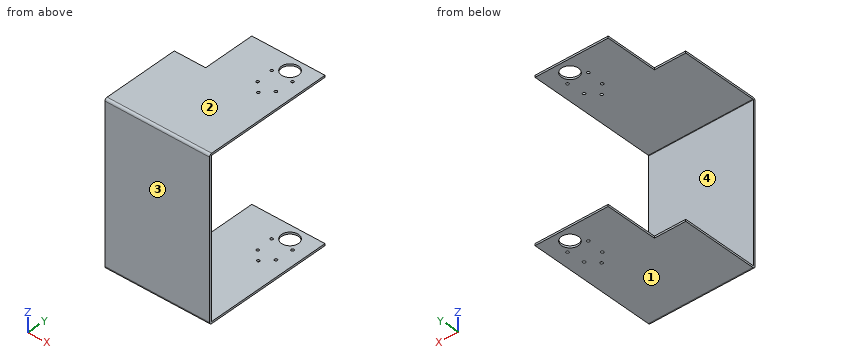
Autodesk Inventor part; units mm, degrees
ref_plane "YZ Plane" through (0, 0, 0) normal (1, 0, 0) x (0, 1, 0)
ref_plane "XZ Plane" through (0, 0, 0) normal (0, 1, 0) x (-1, 0, 0)
ref_plane "XY Plane" through (0, 0, 0) normal (0, 0, 1) x (1, 0, 0)
sketch "Sketch1" plane through (0, 0, 0) normal (0, 1, 0) x (-1, 0, 0)
  line L0 (0, 0) -> (80, 0)
  line L1 (80, 0) -> (80, 120)
  line L2 (80, 120) -> (0, 120)
  line L3 (0, 120) -> (0, 0)
  dimension "d0" = 80
  dimension "d1" = 120
extrude "Plate1" add sketch "Sketch1" along normal blind 1.5
sketch "Sketch2" plane through (0, 0, 121.5) normal (0, 0, -1) x (-1, 0, 0)
  line L0 (80, 0) -> (0, 0)
  line L1 (0, 0) -> (0, 100)
  line L2 (0, 100) -> (80, 100)
  line L3 (80, 100) -> (80, 0)
edge flange "Flange1" height 100 angle 90 thickness 1.5 bend radius 0.31 thickness toward (0, 0, -1) relief tear relief width 1.5 relief depth 0.75 edges at (-40, 1.5, 120) wall of the first edge with corners at (-80, 0, 121.5) (0, 0, 121.5) (0, 100, 121.5) (-80, 100, 121.5)
bend "Bend1"
corner "Corner1"
sketch "Sketch3" plane through (-80, 0, -1.5) normal (0, 0, 1) x (1, 0, 0)
  line L0 (80, 0) -> (0, 0)
  line L1 (0, 0) -> (0, 100)
  line L2 (0, 100) -> (80, 100)
  line L3 (80, 100) -> (80, 0)
edge flange "Flange2" height 100 angle 90 thickness 1.5 bend radius 0.31 thickness toward (0, 0, 1) relief tear relief width 1.5 relief depth 0.75 edges at (-40, 1.5, 0) wall of the first edge with corners at (0, 0, -1.5) (-80, 0, -1.5) (-80, 100, -1.5) (0, 100, -1.5)
bend "Bend2"
corner "Corner2"
sketch "Sketch4" plane through (0, 100, -1.5) normal (0, 0, -1) x (-1, 0, 0)
  line L0 (56, -40) -> (80, -40)
  line L1 (80, -40) -> (80, 0)
  line L2 (80, 0) -> (56, 0)
  line L3 (56, 0) -> (56, -40)
  line L4 (80, 0) -> (80, -98.19)
  line L5 (0, 0) -> (80, 0)
  point P0 (0, -100)
  dimension "d23" = 24
  dimension "d24" = 40
extrude "Cut1" cut sketch "Sketch4" against normal blind 1.5
sketch "Sketch5" plane through (0, 100, 120) normal (0, 0, -1) x (-1, 0, 0)
  point P0 (0, -100)
sketch "Sketch6" plane through (-80, 100, 121.5) normal (0, 0, 1) x (1, 0, 0)
  line L0 (24, 0) -> (0, 0)
  line L1 (0, 0) -> (0, -40)
  line L2 (0, -40) -> (24, -40)
  line L3 (24, -40) -> (24, 0)
  line L4 (0, -98.19) -> (0, 0)
  line L5 (0, 0) -> (80, 0)
  point P0 (80, -100)
  dimension "d27" = 40
  dimension "d28" = 24
extrude "Cut2" cut sketch "Sketch6" against normal blind 1.5
sketch "Sketch7" plane through (0, 1.81, -1.5) normal (0, 0, -1) x (-1, 0, 0)
  circle A0 centre (17.93, 60.77) radius 0.7835
  circle A1 centre (10.93, 68.07) radius 0.7835
  circle A2 centre (24.93, 68.07) radius 0.7835
  circle A3 centre (9.93, 81.29) radius 0.7835
  circle A4 centre (25.93, 81.29) radius 0.7835
  line L0 (24, 59.37) -> (11.86, 59.37)
  line L1 (24, 59.37) -> (24, 60.09)
  arc A5 (26, 62.09) -> (24, 60.09) centre (26, 60.09) ccw
  line L2 (26, 62.09) -> (26.72, 62.09)
  line L3 (26.72, 94.19) -> (26.72, 62.09)
  line L4 (26.72, 94.19) -> (26, 94.19)
  arc A6 (24, 96.19) -> (26, 94.19) centre (26, 96.19) ccw
  line L5 (24, 96.19) -> (24, 96.91)
  line L6 (11.86, 96.91) -> (24, 96.91)
  line L7 (11.86, 96.91) -> (11.86, 96.19)
  arc A7 (9.86, 94.19) -> (11.86, 96.19) centre (9.86, 96.19) ccw
  line L8 (9.86, 94.19) -> (9.14, 94.19)
  line L9 (9.14, 62.09) -> (9.14, 94.19)
  line L10 (9.14, 62.09) -> (9.86, 62.09)
  arc A8 (11.86, 60.09) -> (9.86, 62.09) centre (9.86, 60.09) ccw
  line L11 (11.86, 60.09) -> (11.86, 59.37)
  circle A9 centre (17.93, 88.19) radius 6.4
  point P0 (0, -1.81)
  point P1 (11.86, 94.19)
hole "Hole1" at (-10.93, 69.88, -1.5) at (-9.93, 83.1, -1.5) at (-25.93, 83.1, -1.5) at (-24.93, 69.88, -1.5) at (-17.93, 62.58, -1.5) direction (0, 0, 1) diameter 2.1 depth 1.5
sketch "Sketch8" plane through (-80, 1.81, 121.5) normal (0, 0, 1) x (1, 0, 0)
  circle A0 centre (62.07, 60.77) radius 0.7835
  circle A1 centre (55.07, 68.07) radius 0.7835
  circle A2 centre (69.07, 68.07) radius 0.7835
  circle A3 centre (54.07, 81.29) radius 0.7835
  circle A4 centre (70.07, 81.29) radius 0.7835
  line L0 (68.14, 59.37) -> (56, 59.37)
  line L1 (68.14, 59.37) -> (68.14, 60.09)
  arc A5 (70.14, 62.09) -> (68.14, 60.09) centre (70.14, 60.09) ccw
  line L2 (70.14, 62.09) -> (70.86, 62.09)
  line L3 (70.86, 94.19) -> (70.86, 62.09)
  line L4 (70.86, 94.19) -> (70.14, 94.19)
  arc A6 (68.14, 96.19) -> (70.14, 94.19) centre (70.14, 96.19) ccw
  line L5 (68.14, 96.19) -> (68.14, 96.91)
  line L6 (56, 96.91) -> (68.14, 96.91)
  line L7 (56, 96.91) -> (56, 96.19)
  arc A7 (54, 94.19) -> (56, 96.19) centre (54, 96.19) ccw
  line L8 (54, 94.19) -> (53.28, 94.19)
  line L9 (53.28, 62.09) -> (53.28, 94.19)
  line L10 (53.28, 62.09) -> (54, 62.09)
  arc A8 (56, 60.09) -> (54, 62.09) centre (54, 60.09) ccw
  line L11 (56, 60.09) -> (56, 59.37)
  circle A9 centre (62.07, 88.19) radius 6.4
  point P0 (80, -1.81)
  point P1 (56, 94.19)
hole "Hole2" at (-25.93, 83.1, 121.5) at (-9.93, 83.1, 121.5) at (-10.93, 69.88, 121.5) at (-24.93, 69.88, 121.5) at (-17.93, 62.58, 121.5) direction (0, 0, -1) diameter 2.1 depth 1.5
sketch "Sketch9" plane through (-80, 1.81, 121.5) normal (0, 0, 1) x (1, 0, 0)
  circle A0 centre (62.07, 60.77) radius 0.7835
  circle A1 centre (55.07, 68.07) radius 0.7835
  circle A2 centre (69.07, 68.07) radius 0.7835
  circle A3 centre (54.07, 81.29) radius 0.7835
  circle A4 centre (70.07, 81.29) radius 0.7835
  line L0 (68.14, 59.37) -> (56, 59.37)
  line L1 (68.14, 59.37) -> (68.14, 60.09)
  arc A5 (70.14, 62.09) -> (68.14, 60.09) centre (70.14, 60.09) ccw
  line L2 (70.14, 62.09) -> (70.86, 62.09)
  line L3 (70.86, 94.19) -> (70.86, 62.09)
  line L4 (70.86, 94.19) -> (70.14, 94.19)
  arc A6 (68.14, 96.19) -> (70.14, 94.19) centre (70.14, 96.19) ccw
  line L5 (68.14, 96.19) -> (68.14, 96.91)
  line L6 (56, 96.91) -> (68.14, 96.91)
  line L7 (56, 96.91) -> (56, 96.19)
  arc A7 (54, 94.19) -> (56, 96.19) centre (54, 96.19) ccw
  line L8 (54, 94.19) -> (53.28, 94.19)
  line L9 (53.28, 62.09) -> (53.28, 94.19)
  line L10 (53.28, 62.09) -> (54, 62.09)
  arc A8 (56, 60.09) -> (54, 62.09) centre (54, 60.09) ccw
  line L11 (56, 60.09) -> (56, 59.37)
  circle A9 centre (62.07, 88.19) radius 6.4
  circle A10 centre (62.07, 88.19) radius 6.5
  point P0 (80, -1.81)
  point P1 (56, 94.19)
  dimension "d45" = 13
extrude "Extrusion1" cut sketch "Sketch9" against normal blind 1.5 contours A9 | A10
sketch "Sketch10" plane through (0, 1.81, -1.5) normal (0, 0, -1) x (-1, 0, 0)
  circle A0 centre (17.93, 60.77) radius 0.7835
  circle A1 centre (10.93, 68.07) radius 0.7835
  circle A2 centre (24.93, 68.07) radius 0.7835
  circle A3 centre (9.93, 81.29) radius 0.7835
  circle A4 centre (25.93, 81.29) radius 0.7835
  line L0 (24, 59.37) -> (11.86, 59.37)
  line L1 (24, 59.37) -> (24, 60.09)
  arc A5 (26, 62.09) -> (24, 60.09) centre (26, 60.09) ccw
  line L2 (26, 62.09) -> (26.72, 62.09)
  line L3 (26.72, 94.19) -> (26.72, 62.09)
  line L4 (26.72, 94.19) -> (26, 94.19)
  arc A6 (24, 96.19) -> (26, 94.19) centre (26, 96.19) ccw
  line L5 (24, 96.19) -> (24, 96.91)
  line L6 (11.86, 96.91) -> (24, 96.91)
  line L7 (11.86, 96.91) -> (11.86, 96.19)
  arc A7 (9.86, 94.19) -> (11.86, 96.19) centre (9.86, 96.19) ccw
  line L8 (9.86, 94.19) -> (9.14, 94.19)
  line L9 (9.14, 62.09) -> (9.14, 94.19)
  line L10 (9.14, 62.09) -> (9.86, 62.09)
  arc A8 (11.86, 60.09) -> (9.86, 62.09) centre (9.86, 60.09) ccw
  line L11 (11.86, 60.09) -> (11.86, 59.37)
  circle A9 centre (17.93, 88.19) radius 6.4
  circle A10 centre (17.93, 88.19) radius 6.5
  point P0 (0, -1.81)
  point P1 (11.86, 94.19)
  dimension "d48" = 13
extrude "Extrusion2" cut sketch "Sketch10" against normal blind 1.5 contours A9 | A10
equation "\"d25\" = Thickness"
equation "\"d29\" = Thickness"
equation "\"d36\" = Thickness"
equation "\"d43\" = Thickness"
equation "\"d2\" = Thickness"
equation "\"d3\" = BendReliefWidth"
equation "\"d4\" = BendReliefDepth"
equation "\"d5\" = MinimumRemnant"
equation "\"d6\" = TransitionRadius"
equation "\"d9\" = BendRadius"
equation "\"d10\" = CornerReliefSize"
equation "\"d11\" = GapSize"
equation "\"d12\" = JacobiRadiusSize"
equation "\"d13\" = BendReliefWidth"
equation "\"d14\" = BendReliefDepth"
equation "\"d15\" = MinimumRemnant"
equation "\"d16\" = TransitionRadius"
equation "\"d19\" = BendRadius"
equation "\"d20\" = CornerReliefSize"
equation "\"d21\" = GapSize"
equation "\"d22\" = JacobiRadiusSize"
equation "\"BendReliefWidth\" = Thickness"
equation "\"BendReliefDepth\" = 0.5 * Thickness"
equation "\"CornerReliefSize\" = 4 * Thickness"
equation "\"MinimumRemnant\" = 2 * Thickness"
equation "\"TransitionRadius\" = BendRadius"
equation "\"JacobiRadiusSize\" = BendRadius"
equation "\"GapSize\" = Thickness"
properties part number "body_main_frame" material "Aluminum 6061-AHC"
Input: part model. Units: mm. Frame: model coordinates. Face numbers are marked on the shaded views. Give positions to 0.01 mm unless a question says otherwise; leave off trailing zeros. Order: outer loops, then holes, each group sorted by start corner. A loop starts at its lowest first (then second) coordinate and runs counter-clockwise, first axis right, second up. Notation, with made-up numbers: (67.5, 86.25) -> (116.5, 86.25) arc R20 cw to (116.5, 112.25) -> close; hole circle Ø6 at (-18.5, 42). An arc over 180 degrees is marked (long way). Write each question's results on one line, items separated by ' | '. Start each with the question number.
Item 1: Contact query for flat-ended pins moving along their axis: P1, Ø12, axis at x = -51, z = 47.5, coming from the +Y side; P2, Ø1.9, axis at x = -25.93, y = 83.1, coming from the +Z side; P3, Ø1.2, axis at y = 83.5, z = -1, coming from the -X side; P4, Ø1.2, axis at x = -73, z = -1, coming from the +Y side. Output: stop coordinate, or through.
Item 2: Cut plane D-D on y = 6. Return the cut outline in (x, z).
Item 3: Cut plane C-C on x = -28.5. Return the cut outline in (y, z).
Item 4: Line query: line 1 (Z direction, x = -39, y = 59); line 2 (X direction, y = 69.88, z = -0.25); line 3 (X direction, y = 83.1, z = 120.8). Output: solid intervals per line, ascending.
Item 5: Mould query, pull axis Z, two halves, no side actions, for the marked faces 1, 2, 3 and 4. Classes: pulls with the +Z half, pulls with the -Z half, needs draft (parallel to the pull), parting line crosses it, or undercut.
Item 6: Cut plane A-A on y = 76.5. Return the cut outline in (x, z), then the cut area to 3 significant figures.
Item 7: Cut plane B-B on y = 90. Return the cut outline in (x, z), then the cut area to 3 significant figures.
Established:
1) P1: y = 1.5 | P2: through | P3: x = -56 | P4: y = 60
2) outline: (-80, -1.5) -> (0, -1.5) -> (0, 0) -> (-80, 0) -> close; (-80, 120) -> (0, 120) -> (0, 121.5) -> (-80, 121.5) -> close
3) outline: (0, 0.31) arc R1.81 ccw to (1.81, -1.5) -> (100, -1.5) -> (100, 0) -> (1.81, 0) arc R0.31 cw to (1.5, 0.31) -> (1.5, 119.69) arc R0.31 cw to (1.81, 120) -> (100, 120) -> (100, 121.5) -> (1.81, 121.5) arc R1.81 ccw to (0, 119.69) -> close
4) line 1: -1.5 to 0, 120 to 121.5 | line 2: -56 to -25.98, -23.88 to -11.98, -9.88 to 0 | line 3: -56 to -26.98, -24.88 to -10.98, -8.88 to 0
5) face 1: pulls with the -Z half | face 2: pulls with the +Z half | face 3: needs draft | face 4: undercut
6) outline: (-56, -1.5) -> (0, -1.5) -> (0, 0) -> (-56, 0) -> close; (-56, 120) -> (0, 120) -> (0, 121.5) -> (-56, 121.5) -> close | area: 168 mm^2
7) outline: (-56, -1.5) -> (-24.43, -1.5) -> (-24.43, 0) -> (-56, 0) -> close; (-56, 120) -> (-24.43, 120) -> (-24.43, 121.5) -> (-56, 121.5) -> close; (-11.43, -1.5) -> (0, -1.5) -> (0, 0) -> (-11.43, 0) -> close; (-11.43, 120) -> (0, 120) -> (0, 121.5) -> (-11.43, 121.5) -> close | area: 129 mm^2
